from build123d import *

# Parameters (mm, degrees)
EXTRUDE_1_DEPTH = 9
EXTRUDE_2_DEPTH = 10


with BuildPart() as part:
    # Эскиз1 → Повернуть1 (revolve)
    with BuildSketch(Plane.XY, mode=Mode.PRIVATE) as revolve_1_sk:
        Polygon((0, 0), (-40, 0), (-40, 16), (-30, 26), (-17, 26), (-17, 29), (-6, 29), (-6, 38), (-6, 136.4), (-4.4, 138), (0, 138), align=None)
    revolve(revolve_1_sk.sketch.rotate(Axis((0, 0, 0), (0, 1, 0)), 180), axis=Axis((0, 0, 0), (0, 1, 0)))  # turned: the seam where the file's is

    # Эскиз2 → Бобышка-Вытянуть1 (add)
    with BuildSketch(Plane(origin=(0, 29, 0), x_dir=(1, 0, 0), z_dir=(0, 1, 0))):
        Polygon((0, 10.969655115), (-9.5, 5.484827557), (-9.5, -5.484827557), (0, -10.969655115), (9.5, -5.484827557), (9.5, 5.484827557), align=None)
    extrude(amount=EXTRUDE_1_DEPTH)

    # Эскиз3 → Бобышка-Вытянуть2 (add)
    with BuildSketch(Plane(origin=(0, 87.2, 0), x_dir=(1, 0, 0), z_dir=(0, 1, 0))):
        Polygon((9.5, 5.484827557), (0, 10.969655115), (-9.5, 5.484827557), (-9.5, -5.484827557), (0, -10.969655115), (9.5, -5.484827557), align=None)
    extrude(amount=EXTRUDE_2_DEPTH)

    # Эскиз4 → Вырез-Повернуть2 (revolve, cut)
    with BuildSketch(Plane.XY, mode=Mode.PRIVATE) as cut_revolve_2_sk:
        Polygon((-18.160254038, 97.2), (-9.5, 97.2), (-18.160254038, 92.2), align=None)
        Polygon((-18.160254038, 87.2), (-18.160254038, 92.2), (-9.5, 87.2), align=None)
        Polygon((-17.294228634, 38), (-17.294228634, 33.5), (-9.5, 38), align=None)
        Polygon((-17.294228634, 33.5), (-17.294228634, 29), (-9.5, 29), align=None)
    revolve(cut_revolve_2_sk.sketch.rotate(Axis((0, 138, 0), (0, -1, 0)), 180), axis=Axis((0, 138, 0), (0, -1, 0)), mode=Mode.SUBTRACT)  # turned: the seam where the file's is


solid = part.part
For this review, take the finished solid that the model builds, in its own axes (mm). A direction names the side the tool comes from. Round coordinates to 2 decimals unless told otherwise and drop trailing zeros. Write each loop counter-clockwise with the first axis right and the second up, starting at its lowest first coordinate (ties: lowest second). Pieces come first, ordered by that corner, then holes. Notation, with made-up numbers: (51, -32.5) -> (69, -32.5) arc R21 ccw to (69, -17.5) -> close; hole circle Ø5 at (-13.5, 28.25). An arc over 180 degrees is marked (long way). Put each result on its own line as item: value.
Q1. Clearance check with flat-ended pins moving along their axes: pin 1 Ø8 at (y, z) = (90.5, 2) entering from -X; pin 2 Ø12 at (x, z) = (-17.5, 27) entering from +Y; pin 3 Ø10 at (x, z) = (5.5, -3.5) entering from +Y; pin 4 Ø5 at (y, z) = (92.5, -2) entering from +X. State where each tip first meets the part, or that it passes through.
Determined:
pin 1: stops at x = -9.5
pin 2: stops at y = 26
pin 3: stops at y = 138
pin 4: stops at x = 9.5
Q2. Consider section A-A on y = 94. State the section outline as (x, z) points, and give its area (3 significant figures).
Determined:
outline: (-9.5, -5.48) -> (0, -10.97) -> (9.5, -5.48) -> (9.5, 5.48) -> (0, 10.97) -> (-9.5, 5.48) -> close
area: 313 mm^2
Q3. Consider section B-B on y = 24. State the section outline as (x, z) points, and give its area (3 significant figures).
Determined:
outline: circle Ø64 at (0, 0)
area: 3,220 mm^2
Q4. To check wall thickness, follow L1, parallel to Y at x = 21, z = -1; L2, parallel to Y at x = 2, z = -16; L3, parallel to Y at x = -1, z = 6. State the ranges of each line that lie inside material, in increasing order. Write a range as [from, to].
Determined:
L1: y = [0, 26]
L2: y = [0, 29]
L3: y = [0, 38], [87.2, 97.2]
Q5. Machinability: for faces 1 (the conical face through (-0.02, 87.4, -9.85)), 2 (the conical face through (-8.519, 37.798, 4.946)), 3 (the flat face through (9.5, 92, 0)), 4 (the flat face through (-0.1, 38, 6.2)), 5 (the cylindrical face through (-2.213, 27.521, -16.855)), which of the approach directions +Z, -Z, +X, -X, +Y, -Y give a long, thin tool a straight path to every point of the face, cutting with its end or side? Answer none if there is none.
Determined:
face 1: -Z
face 2: +Z, -X
face 3: +Z, -Z, +X, +Y
face 4: none
face 5: +Y
